Source: three-view drawing plus pictorial views. Frame: mm from the lowest corner of the part. A direction names the side the tool comes from. Give positions to 0.01 mm unless a question says otherwise; leave off trailing zeros. Order: outer loops, then holes, each group sorted by start corner. A loop starts at its lowest first (then second) coordinate and runs counter-clockwise, first axis right, second up. Notation, with made-up numbers: M 3,-17 L 49,-17 A22 ccw 49,-3 Z; hole C 87.5,67.5 d3. An arc over 180 degrees is marked long. One line per item, written item: value. Start each with the question number.
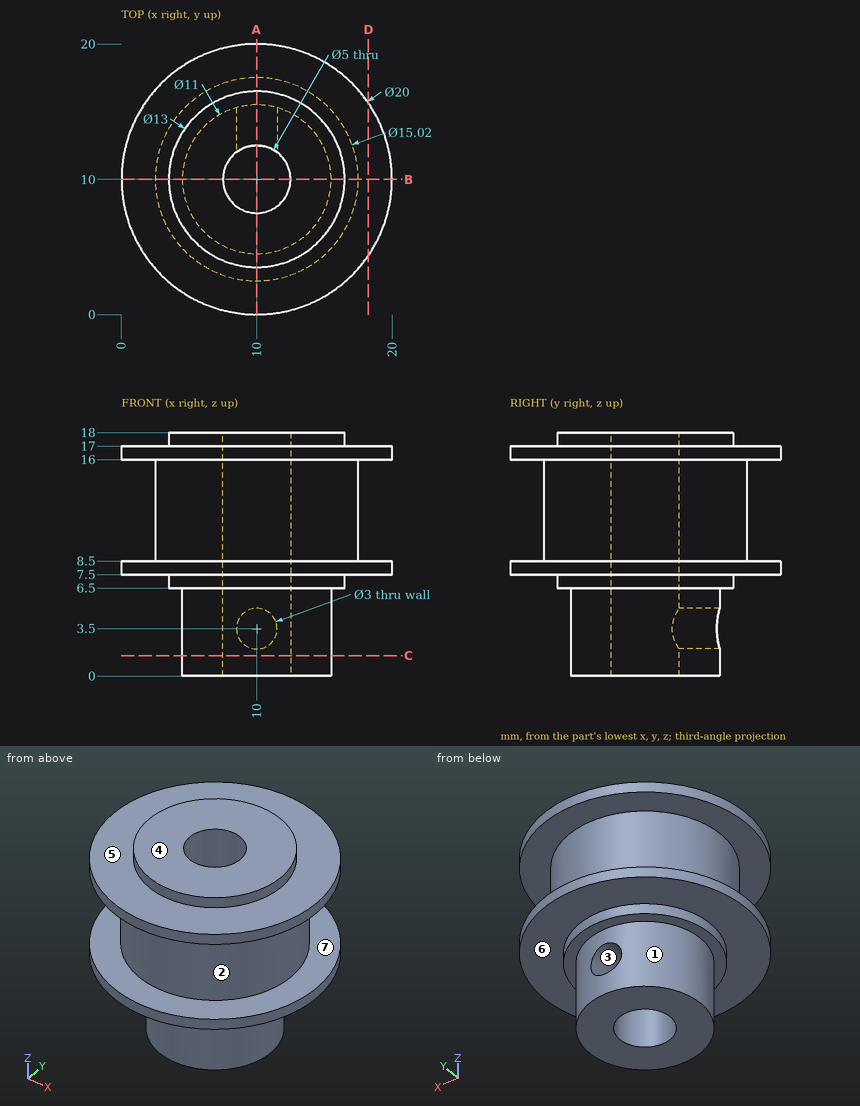
Q1. Contact query for flat-ended pins moving along their axis: pin 1 (1 mm diameter, centred on x = 11.5, z = 10.5, fed in from -Y); pin 2 (8 mm diameter, centred on x = 4, z = 14.5, fed in from -Y); pin 3 (2.5 mm diameter, centred on x = 10, z = 3.5, fed in from -Y). Output: stop coordinate, or through.
Q2. Set-up query: the marked faces 1, 2, 3 and 4. Return all of +Z, -Z, +X, -X, +Y, -Y with unobstructed straight access to the full face (end or side cutting, diameter ignored); none if empty.
Q3. Section query C-C on z = 1.5. Return loops of the section in (x, y), and give its area (3 significant figures).
Q4. Section query B-B on y = 10. Return loops of the section in (x, z), and give its area (3 significant figures).
Q5. Ray query, line 1 along Z through (x, y) = (10, 13.85); line 2 along Z through (x, y) = (2.25, 10.25); line 3 along Y through (x, z) = (10, 7). Return the intervals inside material, ascending. Write a range as [from, to].
Q6. Section query A-A on x = 10. Give the number of separate pieces and of enclosed holes in the cut face, and give its area (3 significant figures).
Q7. Section query D-D on x = 18.25. Return loops of the section in (y, z), and give its area (3 significant figures).
Q8. Mould query, pull axis Z, two halves, no side actions, for the marked faces 5, 6 and 7. Classes: +Z half, -Z half, draft (parallel to the pull), parting line (faces both ways), or undercut.
Results below:
1. pin 1: y = 2.56
1. pin 2: y = 0.27
1. pin 3: y = 4.5
2. face 1: -Z
2. face 2: none
2. face 3: +Y
2. face 4: +Z, +X, -X, +Y, -Y
3. outline: C 10,10 d11; hole C 10,10 d5
3. area: 75.4 mm2
4. outline: M 0,7.5 L 3.5,7.5 L 3.5,6.5 L 4.5,6.5 L 4.5,0 L 7.5,0 L 7.5,18 L 3.5,18 L 3.5,17 L 0,17 L 0,16 L 2.49,16 L 2.49,8.5 L 0,8.5 Z; M 12.5,0 L 15.5,0 L 15.5,6.5 L 16.5,6.5 L 16.5,7.5 L 20,7.5 L 20,8.5 L 17.51,8.5 L 17.51,16 L 20,16 L 20,17 L 16.5,17 L 16.5,18 L 12.5,18 Z
4. area: 160 mm2
5. line 1: [0, 2], [5, 18]
5. line 2: [7.5, 8.5], [16, 17]
5. line 3: [3.5, 7.5], [12.5, 16.5]
6. separate pieces: 3
6. enclosed holes: 0
6. area: 151 mm2
7. outline: M 4.35,7.5 L 15.65,7.5 L 15.65,8.5 L 4.35,8.5 Z; M 4.35,16 L 15.65,16 L 15.65,17 L 4.35,17 Z
7. area: 22.6 mm2
8. face 5: +Z half
8. face 6: -Z half
8. face 7: undercut
